Could you check a few things on this model? Use its own coordinates, in mm. A direction names the side the tool comes from. Coordinates: 2 decimals unless noted, no trailing zeros. Order: outer loops, then holes, each group sorted by start corner. A loop starts at its lowest first (then second) coordinate and runs counter-clockwise, first axis right, second up. Notation, with made-up numbers: (69, 4) - (107, 4) arc R9 cw to (107, 10) - close; hole circle Ø11 at (19.25, 14.25). An arc over 180 degrees is marked (long way). One line per item, written item: value. Start each with the question number.
from build123d import *

# Parameters (mm, degrees)
F2_R     = 2
F3_DEPTH = 10
F5_START = -0.5
F5_DEPTH = 2.501
F6_SIZE2 = 1
F6_SIZE  = 2
F7_R     = 0.5


with BuildPart() as f1:
    # F0 (on Front) → F1 (revolve)
    with BuildSketch(Plane.XZ):
        with BuildLine():
            Line((0, 0), (0, 3))
            ThreePointArc((0, 3), (-2.7041634566, 2.1812451849), (-4.5, 0))
            Line((-4.5, 0), (0, 0))
        make_face()
    revolve(axis=Axis((0, 0, 1.5), (0, 0, -1)))

    # F2 (on face) → F3 (join)
    with BuildSketch(Plane(origin=(0, 0, 0), x_dir=(1, 0, 0), z_dir=(0, 0, -1))):
        Circle(F2_R)
    extrude(amount=F3_DEPTH)

    # F4 (on face) → F5 (cut)
    with BuildSketch(Plane(origin=(0, 0, 0), x_dir=(1, 0, 0), z_dir=(0, 0, -1)).offset(F5_START)):
        Polygon((0.55, 2.05), (0, 2.05), (-0.55, 2.05), (-0.55, 0.55), (-2.05, 0.55), (-2.05, 0), (-2.05, -0.55), (-0.55, -0.55), (-0.55, -2.05), (0, -2.05), (0.55, -2.05), (0.55, -0.55), (2.05, -0.55), (2.05, 0), (2.05, 0.55), (0.55, 0.55), align=None)
    extrude(amount=-F5_DEPTH, mode=Mode.SUBTRACT)

    # F6
    f6_edges = [f1.edges().sort_by_distance(p)[0] for p in [
        (2.05, 0, 0.5),
        (0, 2.05, 0.5),
        (0, -2.05, 0.5),
        (-2.05, 0, 0.5),
    ]]
    chamfer(f6_edges, length=F6_SIZE, length2=F6_SIZE2)

    # F7
    f7_edges = [f1.edges().sort_by_distance(p)[0] for p in [
        (0.55, -0.55, 1.718774),
        (0.55, 0.55, 1.718774),
        (-0.55, -0.55, 1.718774),
        (-0.55, 0.55, 1.718774),
    ]]
    fillet(f7_edges, radius=F7_R)


solid = f1.part
Q1. I want a section at D-D on z = -7.75. Please give me the cut outline in (x, y).
Q2. We'd pull the mould along Y, two halves only. Please class faces 3 (the flat face through (1.4, -0.55, 1.9)), 4 (the cylindrical face through (0, 2, -5)), 5 (the flat face through (-1.543, -0.008, 1.486)), 6 (the flat face through (0, 0, -10)): +Y half, -Y half, draft (parallel to the pull), parting line (faces both ways), or undercut.
Q3. I'm going to push flat-ended pins straight in: pin 1 (0.5 mm diameter, centred on y = -1.5, z = 1, fed in from -X); pin 2 (0.5 mm diameter, centred on y = -1.5, z = 1, fed in from +X); pin 3 (0.5 mm diameter, centred on x = 2, z = 2, fed in from +Y). Where does each tip first touch, or does it pass through?
Q4. If I drill on L1, parallel to Z at x = 2, y = 2.75; L2, parallel to Y at x = -1.25, z = -7.75; L3, parallel to Z at x = -1.5, y = 3, over which ranges is the centre line in solid material (lowest first)?
Q5. Which directions (+Z, -Z, +X, -X, +Y, -Y) give clear straight access to the entire face, cutting with the end or side of a thin tool? Please do faces 1 (the flat face through (-1, -2, 0)), 2 (the flat face through (0.55, -1.4, 1.9)).
Q6. I want a section at B-B on y = 0. Please give me the cut outline in (x, z) (3 decimals).
Q7. I want a section at A-A on z = 1.75. Please give me the cut outline in (x, y) (3 decimals), then the cut area to 3 significant figures.
Values follow:
1. outline: circle Ø4 at (0, 0)
2. face 3: undercut
2. face 4: parting line
2. face 5: undercut
2. face 6: draft
3. pin 1: stops at x = -3.85
3. pin 2: stops at x = 3.85
3. pin 3: stops at y = 2.62
4. L1: z = 0 to 1.62
4. L2: y = -1.56 to 1.56
4. L3: z = 0 to 1.66
5. face 1: -Z
5. face 2: +Z
6. outline: (-4.5, 0) - (-2, 0) - (-2, -10) - (2, -10) - (2, 0) - (4.5, 0) arc R4.875 ccw to (2.05, 2.548) - (2.05, 2.5) - (1.05, 0.5) - (-1.05, 0.5) - (-2.05, 2.5) - (-2.05, 2.548) arc R4.875 ccw to start
7. outline: circle Ø6.519 at (0, 0); hole (-1.675, -0.55) - (-1.05, -0.55) arc R0.5 cw to (-0.55, -1.05) - (-0.55, -1.675) - (0.55, -1.675) - (0.55, -1.05) arc R0.5 cw to (1.05, -0.55) - (1.675, -0.55) - (1.675, 0.55) - (1.05, 0.55) arc R0.5 cw to (0.55, 1.05) - (0.55, 1.675) - (-0.55, 1.675) - (-0.55, 1.05) arc R0.5 cw to (-1.05, 0.55) - (-1.675, 0.55) - close
7. area: 27.0 mm^2
